```python
from build123d import *

# Parameters (mm, degrees)
F1_DEPTH = 2
F2_W     = 5
F2_H     = 2
F3_DEPTH = 25
F4_W     = 5
F4_H     = 2
F5_DEPTH = 25
F6_R     = 12
F7_DEPTH = 25


with BuildPart() as f1:
    # F0 (on Right) → F1 (new body)
    with BuildSketch(Plane.YZ):
        Polygon((60, 46.556178), (0, 46.556178), (-60, 46.556178), (-60, -58.443822), (0, -58.443822), (60, -58.443822), align=None)
    extrude(amount=F1_DEPTH)

    # F2 (on face) → F3 (cut)
    with BuildSketch(Plane.YZ.offset(2)):
        with Locations((-47.5, -47.443822)):
            Rectangle(F2_W, F2_H)
        with Locations((47.5, -47.443822)):
            Rectangle(F2_W, F2_H)
        with Locations((-47.5, -39.443822)):
            Rectangle(F2_W, F2_H)
        with Locations((47.5, -39.443822)):
            Rectangle(F2_W, F2_H)
    extrude(amount=-F3_DEPTH, mode=Mode.SUBTRACT)

    # F4 (on face) → F5 (cut)
    with BuildSketch(Plane.YZ.offset(2)):
        with Locations((-45.5, 8.556178)):
            Rectangle(F4_W, F4_H)
        with Locations((-45.5, 16.556178)):
            Rectangle(F4_W, F4_H)
        with Locations((45.5, 8.556178)):
            Rectangle(F4_W, F4_H)
        with Locations((45.5, 16.556178)):
            Rectangle(F4_W, F4_H)
    extrude(amount=-F5_DEPTH, mode=Mode.SUBTRACT)

    # F6 (on face) → F7 (cut)
    with BuildSketch(Plane.YZ.offset(2)):
        Circle(F6_R)
    extrude(amount=-F7_DEPTH, mode=Mode.SUBTRACT)


solid = f1.part
```
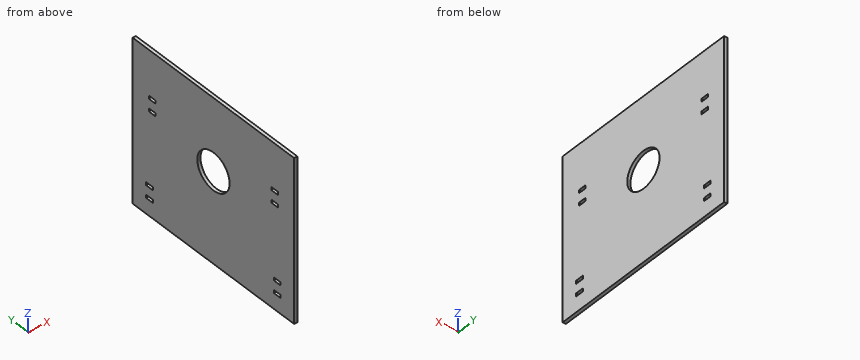
Geometry check sheet. Reference: the model listing, model coordinates, mm. Coordinates: 2 decimals unless noted, no trailing zeros. Order: outer loops, then holes, each group sorted by start corner. A loop starts at its lowest first (then second) coordinate and runs counter-clockwise, first axis right, second up. Notation, with made-up numbers: (62.5, 41) - (69.5, 41) arc R25 ccw to (69.5, 69) - close; hole circle Ø10 at (58.25, 2). An arc over 180 degrees is marked (long way). Answer in a Markdown table with one row per item. Add a question column.
1. Section check A-A (y = 0). Enter the section's corners in (x, z).
2. Section check B-B (z = 0). Enter the section's corners in (x, y), plus the area to 3 significant figures.
3. Section check C-C (x = 0.5). Give the number of separate pieces and of enclosed holes in the cut face, plus the area to 3 significant figures.
4. Material ranges on L1, parallel to Y at x = 1.65, z = -40; L2, parallel to Z at x = 1.2, y = 0; L3, parallel to Z at x = 0.7, y = 11, recorded low to high. Write a range as [from, to].
Data:
| question | item | result |
|---|---|---|
| 1 | outline | (0, -58.44) - (2, -58.44) - (2, -12) - (0, -12) - close; (0, 12) - (2, 12) - (2, 46.56) - (0, 46.56) - close |
| 2 | outline | (0, -60) - (2, -60) - (2, -12) - (0, -12) - close; (0, 12) - (2, 12) - (2, 60) - (0, 60) - close |
| 2 | area | 192 mm² |
| 3 | separate pieces | 1 |
| 3 | enclosed holes | 9 |
| 3 | area | 12,100 mm² |
| 4 | L1 | y = [-60, -50], [-45, 45], [50, 60] |
| 4 | L2 | z = [-58.44, -12], [12, 46.56] |
| 4 | L3 | z = [-58.44, -4.8], [4.8, 46.56] |
